Could you check a few things on this model? Use its own coordinates, in mm. A direction names the side the tool comes from. Give positions to 0.01 mm unless a question says otherwise; leave off trailing zeros. Loops run counter-clockwise (first coordinate to the right, second up) from the corner with the lowest first, then second, coordinate; pieces in that order, holes last. Notation, with made-up numbers: M 78.5,56.5 L 128.5,56.5 A19 cw 128.5,83.5 Z; hole C 7,-35.5 d5. An arc over 180 degrees is marked long. Return JSON: item names as keys, results as strings. Group by question number.
1. For faces 1 (the flat face through (-3, -6, -1)), 2 (the flat face through (11.5, 1, 0)), 3 (the cylindrical face through (4.5, -3, -0.1)), which set-ups out of +Z, -Z, +X, -X, +Y, -Y let a thin tool reach every point of the face, with its end or its side?
2. If we section it at A-A (x = 14): Write out the boundary of the cut face in (y, z), plus the area to 3 significant figures.
3. If we section it at D-D (y = 13.5): Write out the boundary of the cut face in (x, z), plus the area to 3 significant figures.
4. If we section it at B-B (z = 4.25): Write out the boundary of the cut face in (x, y), plus the area to 3 significant figures.
5. If we section it at C-C (x = -11): Write out the boundary of the cut face in (y, z), plus the area to 3 significant figures.
6. Please list where these lines run through material, in increasing order: line 1 (Z direction, x = -14, y = 2.95); line 2 (X direction, y = 3.6, z = 0); line 3 (Y direction, x = 14, z = 5.75).
7. For pin 1 (2 mm diameter, centred on x = 14, z = -0.5, fed in from -Y); pin 2 (1 mm diameter, centred on y = 15.5, z = -3.5, fed in from -X); pin 3 (1.5 mm diameter, centred on x = 0.5, y = -4, fed in from -Z); pin 4 (1.6 mm diameter, centred on x = 14, z = 0, fed in from +Y), each with a flat end and sliding along its axis, tell me the tip position at first contact or that it passes through.
8. If we mould it in two halves opening along X, with no side actions, what happens to faces 4 (the cylindrical face through (-11.496, -2.958, 0.224)), 5 (the flat face through (1, -3, 2.75)), 6 (the cylindrical face through (-13, 3, 0))? For each: +X half, -X half, draft (parallel to the pull), parting line (faces both ways), or undercut.
```python
from build123d import *

# Parameters (mm, degrees)
SKETCH_1_W          = 23
SKETCH_1_H          = 12
EXTRUDE_1_DEPTH     = 22.5
SKETCH_3_W          = 32
SKETCH_3_H          = 12
EXTRUDE_2_DEPTH     = 3
CUT_EXTRUDE_1_DEPTH = 3
SKETCH_5_R          = 6
EXTRUDE_3_DEPTH     = 6
SKETCH_6_R          = 2.5
EXTRUDE_4_DEPTH     = 3.5
EXTRUDE_5_DEPTH     = 6
SKETCH_8_W          = 3
SKETCH_8_H          = 0.8
EXTRUDE_6_DEPTH     = 1


with BuildPart() as part:
    # 草图1 → 凸台-拉伸1 (new body)
    with BuildSketch(Plane(origin=(0, 0, 0), x_dir=(1, 0, 0), z_dir=(0, 1, 0))):
        Rectangle(SKETCH_1_W, SKETCH_1_H)
    extrude(amount=EXTRUDE_1_DEPTH)

    # 草图3 → 凸台-拉伸2 (add)
    with BuildSketch(Plane(origin=(0, 4.5, 0), x_dir=(1, 0, 0), z_dir=(0, 1, 0))):
        Rectangle(SKETCH_3_W, SKETCH_3_H)
    extrude(amount=-EXTRUDE_2_DEPTH)

    # 草图4 → 切除-拉伸1 (cut)
    with BuildSketch(Plane.XZ.offset(-1.5)):
        with BuildLine():
            Line((-16.941045567, 0.5), (-14.866025404, 0.5))
            ThreePointArc((-14.866025404, 0.5), (-13, 0), (-14.866025404, -0.5))
            Line((-14.866025404, -0.5), (-16.941045567, -0.5))
            Line((-16.941045567, -0.5), (-16.941045567, 0.5))
        make_face()
        with BuildLine():
            Line((16.941045567, 0.5), (16.941045567, -0.5))
            Line((16.941045567, -0.5), (14.866025404, -0.5))
            ThreePointArc((14.866025404, -0.5), (13, 0), (14.866025404, 0.5))
            Line((14.866025404, 0.5), (16.941045567, 0.5))
        make_face()
    extrude(amount=-CUT_EXTRUDE_1_DEPTH, mode=Mode.SUBTRACT)

    # 草图5 → 凸台-拉伸3 (add)
    with BuildSketch(Plane.XZ):
        with Locations(Location((-5.5, 0, 0), (0, 0, 270))):
            Circle(SKETCH_5_R)
    extrude(amount=EXTRUDE_3_DEPTH)

    # 草图6 → 凸台-拉伸4 (add)
    with BuildSketch(Plane.XZ.offset(6)):
        with Locations(Location((-5.5, 0, 0), (0, 0, 270))):
            Circle(SKETCH_6_R)
    extrude(amount=EXTRUDE_4_DEPTH)

    # 草图7 → 凸台-拉伸5 (add)
    with BuildSketch(Plane(origin=(0, 0, 0), x_dir=(1, 0, 0), z_dir=(0, 1, 0))):
        with BuildLine():
            Line((1.75, -2.75), (-1.67047712, -2.75))
            Line((-1.67047712, -2.75), (-1.67047712, 2.75))
            Line((-1.67047712, 2.75), (1.75, 2.75))
            ThreePointArc((1.75, 2.75), (4.5, 0), (1.75, -2.75))
        make_face()
    extrude(amount=-EXTRUDE_5_DEPTH)

    # 草图8 → 凸台-拉伸6 (add)
    with BuildSketch(Plane.ZY.offset(11.5)):
        with Locations((0, 17.9)):
            Rectangle(SKETCH_8_W, SKETCH_8_H)
    extrude(amount=EXTRUDE_6_DEPTH)


solid = part.part
```
Answer:
{
 "1": {"face 1": "-Y", "face 2": "+Z, -Z, +X, -Y", "face 3": "+X, -Y"},
 "2": {"outline": "M 1.5,-6 L 4.5,-6 L 4.5,-1 L 1.5,-1 Z; M 1.5,1 L 4.5,1 L 4.5,6 L 1.5,6 Z", "area": "30.0 mm²"},
 "3": {"outline": "M -11.5,-6 L 11.5,-6 L 11.5,6 L -11.5,6 Z", "area": "276 mm²"},
 "4": {"outline": "M -16,1.5 L -11.5,1.5 L -11.5,0 L -9.74,0 L -9.74,-6 L -1.26,-6 L -1.26,0 L 11.5,0 L 11.5,1.5 L 16,1.5 L 16,4.5 L 11.5,4.5 L 11.5,22.5 L -11.5,22.5 L -11.5,4.5 L -16,4.5 Z", "area": "595 mm²"},
 "5": {"outline": "M -6,-2.4 L 0,-2.4 L 0,-6 L 22.5,-6 L 22.5,6 L 0,6 L 0,2.4 L -6,2.4 Z", "area": "299 mm²"},
 "6": {"line 1": "z = -6 to -1, 1 to 6", "line 2": "x = -13 to 13", "line 3": "y = 1.5 to 4.5"},
 "7": {"pin 1": "stops at y = 1.5", "pin 2": "stops at x = -11.5", "pin 3": "stops at z = -2.9", "pin 4": "passes through"},
 "8": {"face 4": "parting line", "face 5": "draft", "face 6": "undercut"}
}
